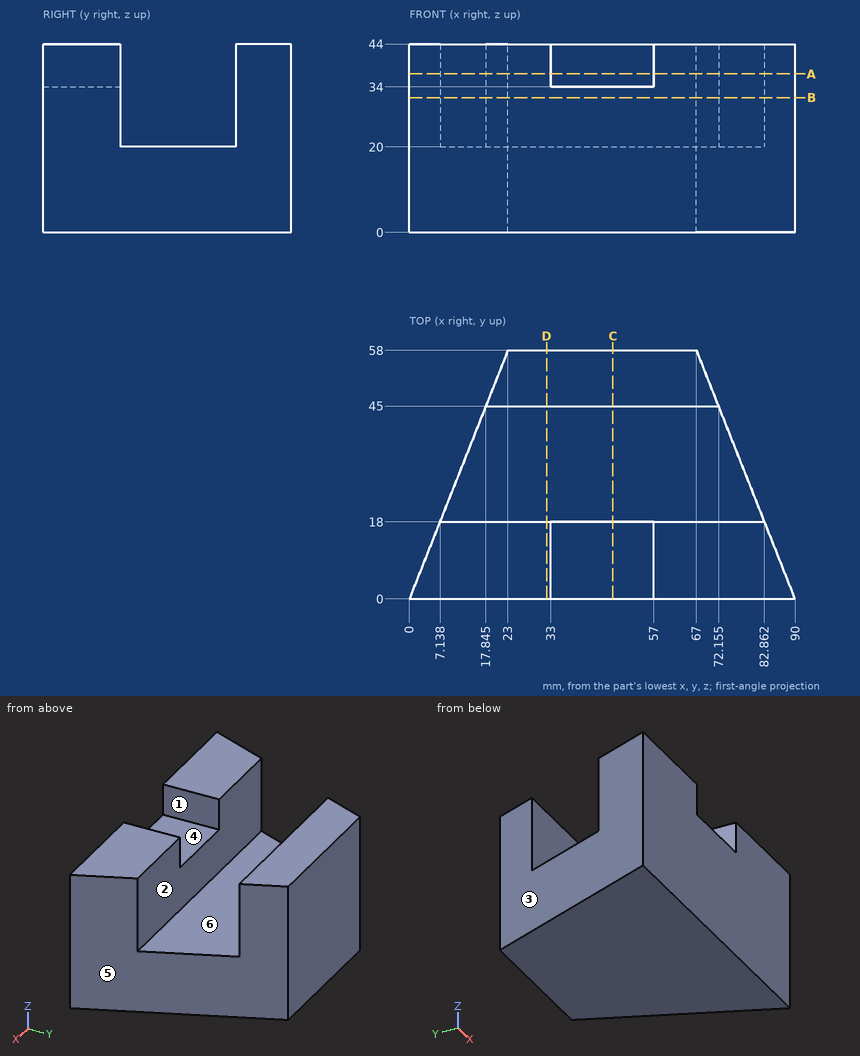
Answer from the drawing. Dimensions are ordinates in mm from the lowest x, y and z of the part. A direction names the side the tool comes from. Give positions to 0.01 mm unless a question says otherwise; leave off trailing zeros. Order: outer loops, then holes, each group sorted by start corner. A loop starts at its lowest first (then second) coordinate and runs counter-clockwise, first axis right, second up. Notation, with made-up numbers: (44, -38) -> (86, -38) arc R15 cw to (86, -20) -> close; hole circle Ø5 at (89, 83.5). An arc over 180 degrees is marked (long way). One line per item, written item: value. Start each with the question number.
(1) The part is cut by section C-C (x = 47.5). Determine the outline of the cut face in (y, z).
(2) The part is cut by section A-A (z = 37). Determine the outline of the cut face in (x, y) (1 decimal), and give its area (3 significant figures).
(3) Flat-ended cylindrical pins translate along their axes: P1, Ø5, axis at y = 5, z = 39.5, coming from the -X side; P2, Ø6, axis at x = 56, y = 34, coming from the +Z side; P3, Ø8, axis at y = 7, z = 40.5, coming from the +X side. Find the tip coordinate at first contact, or state that the pin passes through.
(4) Straight lines are drawn through the part: L1, parallel to Y at x = 47, z = 36; L2, parallel to Z at x = 41.5, y = 26; L3, parallel to Y at x = 79, z = 25. For each, find the intervals that lie inside material, in ascending order.
(5) For a pull along X with two mould halves and no side action, classify the marked faces 1, 2 and 3 as released by +X, released by -X, zero draft, split by the parting line, or undercut.
(6) The part is cut by section B-B (z = 31.5). Determine the outline of the cut face in (x, y) (1 decimal), and give its area (3 significant figures).
(7) The part is cut by section D-D (x = 32). Determine the outline of the cut face in (y, z).
(8) A tool of negligible diameter and unlimited length cuts with its end or side. For the marked faces 4, 5 and 6, from which of +Z, -Z, +X, -X, +Y, -Y can it reach the whole face along a straight path? Write none if from no direction.
Taken from the geometry:
1. outline: (0, 0) -> (58, 0) -> (58, 44) -> (45, 44) -> (45, 20) -> (18, 20) -> (18, 34) -> (0, 34) -> close
2. outline: (0, 0) -> (33, 0) -> (33, 18) -> (7.1, 18) -> close; (17.8, 45) -> (72.2, 45) -> (67, 58) -> (23, 58) -> close; (57, 0) -> (90, 0) -> (82.9, 18) -> (57, 18) -> close
2. area: 1,700 mm^2
3. P1: x = 0.99
3. P2: z = 20
3. P3: x = 88.81
4. L1: 45 to 58
4. L2: 0 to 20
4. L3: 0 to 18
5. face 1: undercut
5. face 2: zero draft
5. face 3: released by -X
6. outline: (0, 0) -> (90, 0) -> (82.9, 18) -> (7.1, 18) -> close; (17.8, 45) -> (72.2, 45) -> (67, 58) -> (23, 58) -> close
6. area: 2,130 mm^2
7. outline: (0, 0) -> (58, 0) -> (58, 44) -> (45, 44) -> (45, 20) -> (18, 20) -> (18, 44) -> (0, 44) -> close
8. face 4: +Z, -Y
8. face 5: +Z, -Z, +X, +Y
8. face 6: +Z, +X, -X
